For this review, take the finished solid that the model builds, in its own axes (mm). A direction names the side the tool comes from. Give positions to 0.01 mm unless a question says otherwise; leave off trailing zeros. Loops run counter-clockwise (first coordinate to the right, second up) from the corner with the lowest first, then second, coordinate; pieces in that order, holes last. Notation, with made-up numbers: (64, 78) - (115, 78) arc R12 ccw to (115, 92) - close; hole circle Ø9 at (85.5, -7.75). An arc over 180 degrees is marked (long way). Put each result on its own line as item: value.
from build123d import *

# Parameters (mm, degrees)
SKETCH_1_R                   = 6
EXTRUDE_1_DEPTH              = 116
HOLE_WIZARD_M3_3_D           = 2.5
HOLE_WIZARD_M3_3_DEPTH       = 6.748924226
HOLE_WIZARD_M3_3_CSINK_D     = 3.05
HOLE_WIZARD_M3_3_CSINK_ANGLE = 45
HOLE_WIZARD_M3_3_TIP         = 0.751075774
HOLE_WIZARD_M3_4_D           = 2.5
HOLE_WIZARD_M3_4_DEPTH       = 6.748924226
HOLE_WIZARD_M3_4_CSINK_D     = 3.05
HOLE_WIZARD_M3_4_CSINK_ANGLE = 45
HOLE_WIZARD_M3_4_TIP         = 0.751075774


with BuildPart() as part:
    # 草圖1 → 填料-伸長1 (new body)
    with BuildSketch(Plane.XY):
        Circle(SKETCH_1_R)
    extrude(amount=EXTRUDE_1_DEPTH)

    # M3 螺紋孔3
    with Locations(Plane.XY.offset(116)):
        with Locations((0, 0)):
            CounterSinkHole(HOLE_WIZARD_M3_3_D / 2, HOLE_WIZARD_M3_3_CSINK_D / 2, depth=HOLE_WIZARD_M3_3_DEPTH, counter_sink_angle=HOLE_WIZARD_M3_3_CSINK_ANGLE)
            with Locations((0, 0, -(HOLE_WIZARD_M3_3_DEPTH + HOLE_WIZARD_M3_3_TIP / 2))):  # 118° drill point
                Cone(0, HOLE_WIZARD_M3_3_D / 2, HOLE_WIZARD_M3_3_TIP, mode=Mode.SUBTRACT)

    # M3 螺紋孔4
    with Locations(Plane(origin=(0, 0, 0), x_dir=(-1, 0, 0), z_dir=(0, 0, -1))):
        with Locations((0, 0)):
            CounterSinkHole(HOLE_WIZARD_M3_4_D / 2, HOLE_WIZARD_M3_4_CSINK_D / 2, depth=HOLE_WIZARD_M3_4_DEPTH, counter_sink_angle=HOLE_WIZARD_M3_4_CSINK_ANGLE)
            with Locations((0, 0, -(HOLE_WIZARD_M3_4_DEPTH + HOLE_WIZARD_M3_4_TIP / 2))):  # 118° drill point
                Cone(0, HOLE_WIZARD_M3_4_D / 2, HOLE_WIZARD_M3_4_TIP, mode=Mode.SUBTRACT)


solid = part.part
1) Take a section at C-C on y = -3.25. State the section outline as (x, z) points.
Geometry check:
outline: (-5.04, 0) - (5.04, 0) - (5.04, 116) - (-5.04, 116) - close
2) For faces 1 (the face through (-0.05, -0.21, 108.63)), 2 (the face through (-0.27, -1.22, 3.75)), list the 3-axis set-ups (+Z, -Z, +X, -X, +Y, -Y) from which the entire face can be reached by the end or side of a thin tool; tool diameter is ignored.
Geometry check:
face 1: +Z
face 2: -Z
3) Take a section at B-B on x = -4.75. State the section outline as (y, z) points, and give its area (3 significant figures).
Geometry check:
outline: (-3.67, 0) - (3.67, 0) - (3.67, 116) - (-3.67, 116) - close
area: 850 mm²
4) Draft analysis for pull direction Y (two halves, no side actions). For faces 3 (the face through (0.05, -0.21, 7.37)), 4 (the face through (1.2, -1.2, 0)), 5 (the face through (0.27, -1.22, 112.25)), 6 (the face through (-6, 0, 57)), state which applies: pulls with the +Y half, pulls with the -Y half, needs draft (parallel to the pull), parting line crosses it, or undercut.
Geometry check:
face 3: undercut
face 4: needs draft
face 5: undercut
face 6: parting line crosses it
5) Wall thickness on line 1 (Y direction, x = 0, z = 3.5); line 2 (X direction, y = 4.75, z = 27.5); line 3 (X direction, y = 3.75, z = 79): over which ranges is each line inside the solid? List them lowest first.
Geometry check:
line 1: y = -6 to -1.25, 1.25 to 6
line 2: x = -3.67 to 3.67
line 3: x = -4.68 to 4.68
6) Take a section at A-A on z = 97. State the section outline as (x, y) points.
Geometry check:
outline: circle Ø12 at (0, 0)
7) Insertion check: pin 1 Ø6 at (y, z) = (-4, 95.5) entering from +X; pin 2 Ø2 at (x, y) = (0, 0) entering from -Z. Each pin has a flat end and moves straight along its axis. Give the tip position at first contact, or say it passes through.
Geometry check:
pin 1: stops at x = 5.92
pin 2: stops at z = 6.9
